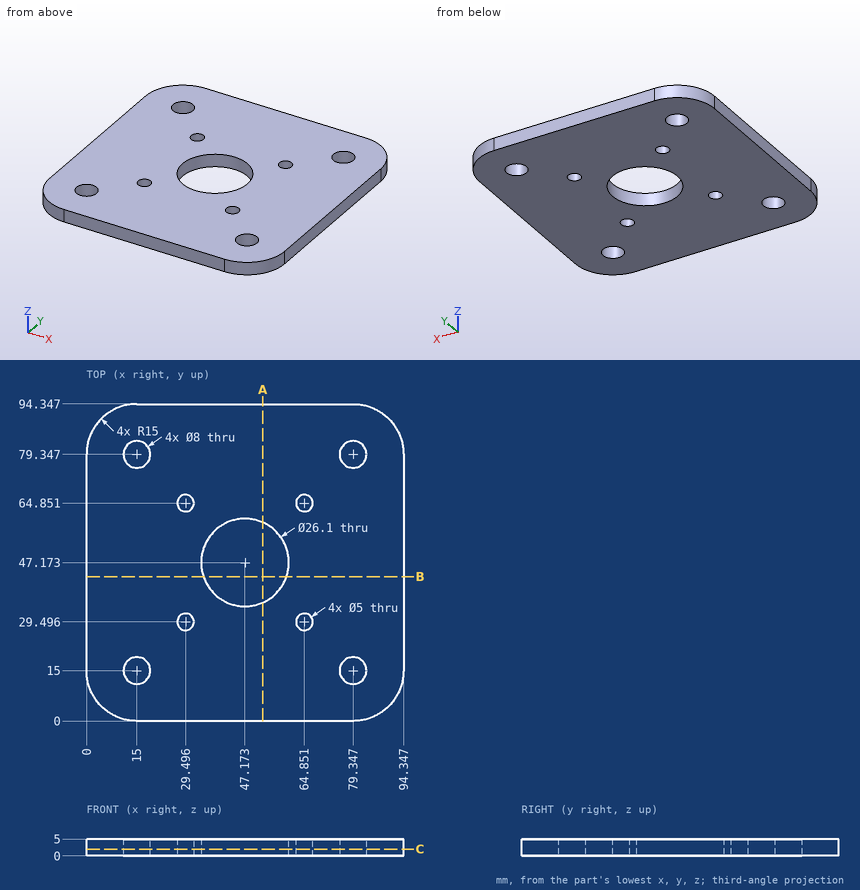
Here's the drawing with two shaded views (mm, measured from the low corner). I have some questions. Coordinates: 2 decimals unless noted, no trailing zeros. Write each loop counter-clockwise with the first axis right and the second up, starting at its lowest first coordinate (ties: lowest second). Pieces come first, ordered by that corner, then holes. Notation, with made-up numbers: M -5.75,-4 L 13.25,-4 A18 ccw 13.25,18 Z; hole C 84.5,66 d4. An arc over 180 degrees is marked long. Answer as CSV lines item,"result". Start each with the question number.
1) For P1, Ø7, axis at x = 15, y = 79.35, coming from the -Z side, with a flat end and sliding along its axis, tell me the tip position at first contact or that it passes through.
2) Please list where these lines run through material, in increasing order: line 1 (Y direction, x = 15, z = 3.5); line 2 (X direction, y = 63, z = 0.5) (1 decimal); line 3 (Y direction, x = 31.5, z = 4.5) (1 decimal). Write a range as from..to.
3) I want a section at C-C, the plane z = 1.95. Give the number of separate pieces and of enclosed holes in the cut face, and give its area (3 significant figures).
4) I want a section at A-A, the plane x = 52.5. Please give me the cut outline in (y, z).
5) I want a section at B-B, the plane y = 43. Please give me the cut outline in (x, z), and give its area (3 significant figures).
Data:
1,P1,"passes through"
2,line 1,"y = 0..11, 19..75.35, 83.35..94.35"
2,line 2,"x = 0..27.8, 31.2..63.2, 66.5..94.3"
2,line 3,"y = 0..28, 31..63.4, 66.3..94.3"
3,separate pieces,"1"
3,enclosed holes,"9"
3,area,"7,890 mm^2"
4,outline,"M 0,0 L 35.26,0 L 35.26,5 L 0,5 Z; M 59.09,0 L 94.35,0 L 94.35,5 L 59.09,5 Z"
5,outline,"M 0,0 L 34.81,0 L 34.81,5 L 0,5 Z; M 59.54,0 L 94.35,0 L 94.35,5 L 59.54,5 Z"
5,area,"348 mm^2"
